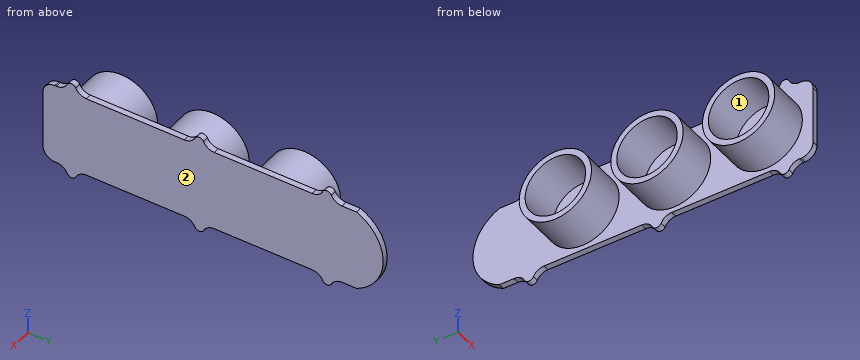
```python
from build123d import *

# Parameters (mm, degrees)
BOSS_EXTRUDE2_START = 50
BOSS_EXTRUDE2_DEPTH = 5
BOSS_EXTRUDE3_START = 55
SKETCH3_R           = 30.5
SKETCH3_R_2         = 25.5
BOSS_EXTRUDE3_DEPTH = 35


# Read off the part's stored shape, not the designer's step: Intersect2
with BuildPart() as part:
    # Sketch2<8> → Boss-Extrude2 (new body)
    with BuildSketch(Plane(origin=(0, 0, 0), x_dir=(0, 0, -1), z_dir=(1, 0, 0)).offset(BOSS_EXTRUDE2_START)):
        with BuildLine():
            Line((-34.5, 78.446358794), (-34.5, 66.149110641))
            ThreePointArc((-34.5, 66.149110641), (-36.048457453, 60.803885802), (-40.214285714, 57.114031612))
            ThreePointArc((-40.214285714, 57.114031612), (-42.5, 53.5), (-40.214285714, 49.885968388))
            ThreePointArc((-40.214285714, 49.885968388), (-36.048457453, 46.196114198), (-34.5, 40.850889359))
            Line((-34.5, 40.850889359), (-34.5, -41.600889359))
            ThreePointArc((-34.5, -41.600889359), (-36.048457453, -46.946114198), (-40.214285714, -50.635968388))
            ThreePointArc((-40.214285714, -50.635968388), (-42.5, -54.25), (-40.214285714, -57.864031612))
            ThreePointArc((-40.214285714, -57.864031612), (-36.048457453, -61.553885802), (-34.5, -66.899110641))
            Line((-34.5, -66.899110641), (-34.5, -149.350889359))
            ThreePointArc((-34.5, -149.350889359), (-36.048457453, -154.696114198), (-40.214285714, -158.385968388))
            ThreePointArc((-40.214285714, -158.385968388), (-42.5, -162), (-40.214285714, -165.614031612))
            ThreePointArc((-40.214285714, -165.614031612), (-36.048457453, -169.303885802), (-34.5, -174.649110641))
            Line((-34.5, -174.649110641), (-34.5, -176))
            ThreePointArc((-34.5, -176), (-31.571067812, -183.071067812), (-24.5, -186))
            Line((-24.5, -186), (24.5, -186))
            ThreePointArc((24.5, -186), (31.571067812, -183.071067812), (34.5, -176))
            Line((34.5, -176), (34.5, -174.649110641))
            ThreePointArc((34.5, -174.649110641), (36.048457453, -169.303885802), (40.214285714, -165.614031612))
            ThreePointArc((40.214285714, -165.614031612), (42.5, -162), (40.214285714, -158.385968388))
            ThreePointArc((40.214285714, -158.385968388), (36.048457453, -154.696114198), (34.5, -149.350889359))
            Line((34.5, -149.350889359), (34.5, -66.899110641))
            ThreePointArc((34.5, -66.899110641), (36.048457453, -61.553885802), (40.214285714, -57.864031612))
            ThreePointArc((40.214285714, -57.864031612), (42.5, -54.25), (40.214285714, -50.635968388))
            ThreePointArc((40.214285714, -50.635968388), (36.048457453, -46.946114198), (34.5, -41.600889359))
            Line((34.5, -41.600889359), (34.5, 40.850889359))
            ThreePointArc((34.5, 40.850889359), (36.048457453, 46.196114198), (40.214285714, 49.885968388))
            ThreePointArc((40.214285714, 49.885968388), (42.5, 53.5), (40.214285714, 57.114031612))
            ThreePointArc((40.214285714, 57.114031612), (36.048457453, 60.803885802), (34.5, 66.149110641))
            Line((34.5, 66.149110641), (34.5, 78.446358794))
            ThreePointArc((34.5, 78.446358794), (0, 100.8), (-34.5, 78.446358794))
        make_face()
    boss_extrude2 = extrude(amount=BOSS_EXTRUDE2_DEPTH)

    # Sketch3 → Boss-Extrude3 (add)
    # profile 1 of 3: a face of its own
    with BuildSketch(Plane(origin=(0, 0, 0), x_dir=(0, 0, -1), z_dir=(1, 0, 0)).offset(BOSS_EXTRUDE3_START)):
        with Locations((0, -146.5)):
            Circle(SKETCH3_R)
        with Locations((0, -146.5)):
            Circle(SKETCH3_R_2, mode=Mode.SUBTRACT)
    # profile 2 of 3: a face of its own
    with BuildSketch(Plane(origin=(0, 0, 0), x_dir=(0, 0, -1), z_dir=(1, 0, 0)).offset(BOSS_EXTRUDE3_START)):
        with Locations((0, -69.25)):
            Circle(SKETCH3_R)
        with Locations((0, -69.25)):
            Circle(SKETCH3_R_2, mode=Mode.SUBTRACT)
    # profile 3 of 3: a face of its own
    with BuildSketch(Plane(origin=(0, 0, 0), x_dir=(0, 0, -1), z_dir=(1, 0, 0)).offset(BOSS_EXTRUDE3_START)):
        with Locations((0, 8)):
            Circle(SKETCH3_R)
        with Locations((0, 8)):
            Circle(SKETCH3_R_2, mode=Mode.SUBTRACT)
    boss_extrude3 = extrude(amount=BOSS_EXTRUDE3_DEPTH)

    # Mirror3: Boss-Extrude2, Boss-Extrude3 across plane
    add(boss_extrude2.mirror(Plane.ZY.offset(-50)))
    add(boss_extrude3.mirror(Plane.ZY.offset(-50)))


with BuildPart() as body_2:
    # Intersect2: the piece on the far side of the plane
    add(part.part)
    split(bisect_by=Plane.YZ.offset(50), keep=Keep.BOTTOM)


with BuildPart() as part_1:
    add(part.part)

    # Intersect2
    split(bisect_by=Plane.YZ.offset(50), keep=Keep.TOP)


solid = body_2.part
```
Could you check a few things on this model? Use its own coordinates, in mm. Face numbers are marked on the shaded views. Coordinates: 2 decimals unless noted, no trailing zeros. Write each loop counter-clockwise with the first axis right and the second up, starting at its lowest first coordinate (ties: lowest second). Pieces come first, ordered by that corner, then holes. Notation, with made-up numbers: M -8.75,66.25 L 31.25,66.25 A32 cw 31.25,104.25 Z; hole C 17,89 d1. An arc over 180 degrees is marked long. Answer as CSV lines item,"result". Start each with the question number.
1) I want a section at D-D, the plane z = -11.5. Please give me the cut outline in (x, y), and give its area (3 significant figures).
2) For P1, Ø1.1, axis at x = 47.5, y = -175.5, coming from the -Z side; P2, Ø12, axis at x = 17.5, z = 21.5, coming from the -Y side; P3, Ø4, axis at x = 47.5, y = -120.5, coming from the +Z side, each with a flat end and sliding along its axis, tell me the tip position at first contact or that it passes through.
3) I want a section at B-B, the plane y = -146.5. Please give me the cut outline in (x, z), and give its area (3 significant figures).
4) Please list where these lines run through material, in increasing order: line 1 (Y direction, x = 17, z = 1); line 2 (Y direction, x = 38, z = -16); line 3 (Z direction, x = 21, y = -146). Write a range as from..to.
5) I want a section at C-C, the plane z = 0. Please give me the cut outline in (x, y).
6) We'd pull the mould along Y, two halves only. Please class the marked faces 1 and 2: +Y half, -Y half, draft (parallel to the pull), parting line (faces both ways), or undercut.
7) I want a section at A-A, the plane x = 42.5. Please give me the cut outline in (y, z), and give its area (3 significant figures).
Data:
1,outline,"M 10,-174.75 L 45,-174.75 L 45,-186 L 50,-186 L 50,99.01 L 45,99.01 L 45,36.25 L 10,36.25 L 10,30.76 L 45,30.76 L 45,-14.76 L 10,-14.76 L 10,-20.25 L 45,-20.25 L 45,-41 L 10,-41 L 10,-46.49 L 45,-46.49 L 45,-92.01 L 10,-92.01 L 10,-97.5 L 45,-97.5 L 45,-118.25 L 10,-118.25 L 10,-123.74 L 45,-123.74 L 45,-169.26 L 10,-169.26 Z"
1,area,"2,580 mm^2"
2,P1,"stops at z = -34.5"
2,P2,"stops at y = -172.77"
2,P3,"stops at z = 34.5"
3,outline,"M 10,-30.5 L 45,-30.5 L 45,-34.5 L 50,-34.5 L 50,34.5 L 45,34.5 L 45,30.5 L 10,30.5 L 10,25.5 L 45,25.5 L 45,-25.5 L 10,-25.5 Z"
3,area,"695 mm^2"
4,line 1,"y = -176.98..-171.98, -121.02..-116.02, -99.73..-94.73, -43.77..-38.77, -22.48..-17.48, 33.48..38.48"
4,line 2,"y = -172.47..-166.36, -126.64..-120.53, -95.22..-89.11, -49.39..-43.28, -17.97..-11.86, 27.86..33.97"
4,line 3,"z = -30.5..-25.5, 25.5..30.5"
5,outline,"M 10,-177 L 45,-177 L 45,-186 L 50,-186 L 50,100.8 L 45,100.8 L 45,38.5 L 10,38.5 L 10,33.5 L 45,33.5 L 45,-17.5 L 10,-17.5 L 10,-22.5 L 45,-22.5 L 45,-38.75 L 10,-38.75 L 10,-43.75 L 45,-43.75 L 45,-94.75 L 10,-94.75 L 10,-99.75 L 45,-99.75 L 45,-116 L 10,-116 L 10,-121 L 45,-121 L 45,-172 L 10,-172 Z"
6,face 1,"undercut"
6,face 2,"draft"
7,outline,"C -146.5,0 d61; C -69.25,0 d61; C 8,0 d61; hole C -146.5,0 d51; hole C -69.25,0 d51; hole C 8,0 d51"
7,area,"2,640 mm^2"
